```python
from build123d import *

# Parameters (mm, degrees)
SKETCH_W        = 56
SKETCH_H        = 56
PAD_DEPTH       = 18.68
PAD001_DEPTH    = 17
SKETCH004_W     = 50
SKETCH004_H     = 50
PAD002_DEPTH    = 3
SKETCH005_W     = 3.539247
SKETCH005_H     = 31.476045
SKETCH005_W_2   = 3.539498
SKETCH005_H_2   = 31.470025
POCKET003_DEPTH = 3
POCKET004_DEPTH = 5
POCKET005_DEPTH = 5
SKETCH003_W     = 10.900068
SKETCH003_H     = 5.909133
SKETCH003_W_2   = 10.899807
SKETCH003_H_2   = 5.880531
POCKET006_DEPTH = 10
POCKET007_DEPTH = 5
SKETCH002_W     = 7.004639
SKETCH002_H     = 5.993783
SKETCH002_W_2   = 50
SKETCH002_H_2   = 4
POCKET008_DEPTH = 5


with BuildPart() as part:
    # Sketch → Pad (new body)
    with BuildSketch(Plane.XY.offset(-11.59)):
        Rectangle(SKETCH_W, SKETCH_H)
        with BuildLine():
            Line((-21.013424, -25), (21.039206, -25))
            ThreePointArc((21.039206, -25), (23.83991, -23.83991), (25, -21.039206))
            Line((25, -21.039206), (25, 21.096275))
            Line((25, 21.096275), (25, 25))
            Line((21.096275, 25), (25, 25))
            Line((21.096275, 25), (-20.979066, 25))
            Line((-20.979066, 25), (-25, 25))
            Line((-25, 20.979066), (-25, 25))
            Line((-25, 20.979066), (-25, -21.013424))
            ThreePointArc((-25, -21.013424), (-23.832359, -23.832359), (-21.013424, -25))
        make_face(mode=Mode.SUBTRACT)
    extrude(amount=PAD_DEPTH)

    # Sketch → Pad001 (join)
    with BuildSketch(Plane.XY.offset(-11.59)):
        Rectangle(SKETCH_W, SKETCH_H)
        with BuildLine():
            Line((-21.013424, -25), (21.039206, -25))
            ThreePointArc((21.039206, -25), (23.83991, -23.83991), (25, -21.039206))
            Line((25, -21.039206), (25, 21.096275))
            Line((25, 21.096275), (25, 25))
            Line((21.096275, 25), (25, 25))
            Line((21.096275, 25), (-20.979066, 25))
            Line((-20.979066, 25), (-25, 25))
            Line((-25, 20.979066), (-25, 25))
            Line((-25, 20.979066), (-25, -21.013424))
            ThreePointArc((-25, -21.013424), (-23.832359, -23.832359), (-21.013424, -25))
        make_face(mode=Mode.SUBTRACT)
    extrude(amount=PAD001_DEPTH)

    # Sketch004 (on Sketch) → Pad002 (join)
    with BuildSketch(Plane.XY.offset(-11.59)):
        Rectangle(SKETCH004_W, SKETCH004_H)
    extrude(amount=PAD002_DEPTH)

    # Sketch005 (on Pad) → Pocket003 (cut)
    with BuildSketch(Plane.XY.offset(-11.59)):
        with Locations((-13.5995, -5.578318)):
            Rectangle(SKETCH005_W, SKETCH005_H)
        with Locations((13.600253, -5.565392)):
            Rectangle(SKETCH005_W_2, SKETCH005_H_2)
    extrude(amount=-POCKET003_DEPTH, mode=Mode.SUBTRACT)

    # Sketch005 (on Pad) → Pocket004 (cut)
    with BuildSketch(Plane.XY.offset(-11.59)):
        with Locations((-13.5995, -5.578318)):
            Rectangle(SKETCH005_W, SKETCH005_H)
        with Locations((13.600253, -5.565392)):
            Rectangle(SKETCH005_W_2, SKETCH005_H_2)
    extrude(amount=-POCKET004_DEPTH, mode=Mode.SUBTRACT)

    # Sketch005 (on Pad) → Pocket005 (cut)
    with BuildSketch(Plane.XY.offset(-11.59)):
        with Locations((-13.5995, -5.578318)):
            Rectangle(SKETCH005_W, SKETCH005_H)
        with Locations((13.600253, -5.565392)):
            Rectangle(SKETCH005_W_2, SKETCH005_H_2)
    extrude(amount=POCKET005_DEPTH, mode=Mode.SUBTRACT)

    # Sketch003 → Pocket006 (cut)
    with BuildSketch(Plane(origin=(25, 0, -3), x_dir=(0, 1, 0), z_dir=(1, 0, 0))):
        with Locations((-8.499979, 4.550172)):
            Rectangle(SKETCH003_W, SKETCH003_H)
        with Locations((8.599925, 4.534825)):
            Rectangle(SKETCH003_W_2, SKETCH003_H_2)
    extrude(amount=POCKET006_DEPTH, mode=Mode.SUBTRACT)

    # Sketch001 → Pocket007 (cut)
    with BuildSketch(Plane(origin=(10, 25, 0.26), x_dir=(1, 0, 0), z_dir=(0, -1, 0))):
        with BuildLine():
            Line((-3.099737, -3.5), (3.104045, -3.5))
            ThreePointArc((3.104045, -3.5), (5.505348, -2.505348), (6.5, -0.104045))
            Line((6.5, -0.104045), (6.5, 0.345505))
            ThreePointArc((6.5, 0.345505), (5.57607, 2.57607), (3.345505, 3.5))
            Line((3.345505, 3.5), (-3.100127, 3.5))
            ThreePointArc((-3.100127, 3.5), (-5.5042, 2.5042), (-6.5, 0.100127))
            Line((-6.5, 0.100127), (-6.5, -0.099737))
            ThreePointArc((-6.5, -0.099737), (-5.504086, -2.504086), (-3.099737, -3.5))
        make_face()
    extrude(amount=-POCKET007_DEPTH, mode=Mode.SUBTRACT)

    # Sketch002 → Pocket008 (cut)
    with BuildSketch(Plane(origin=(0, 25, -3), x_dir=(1, 0, 0), z_dir=(0, -1, 0))):
        with Locations((-8.503573, 4.513289)):
            Rectangle(SKETCH002_W, SKETCH002_H)
        with Locations((-0.011459, 8.993781)):
            Rectangle(SKETCH002_W_2, SKETCH002_H_2)
    extrude(amount=-POCKET008_DEPTH, mode=Mode.SUBTRACT)


solid = part.part
```
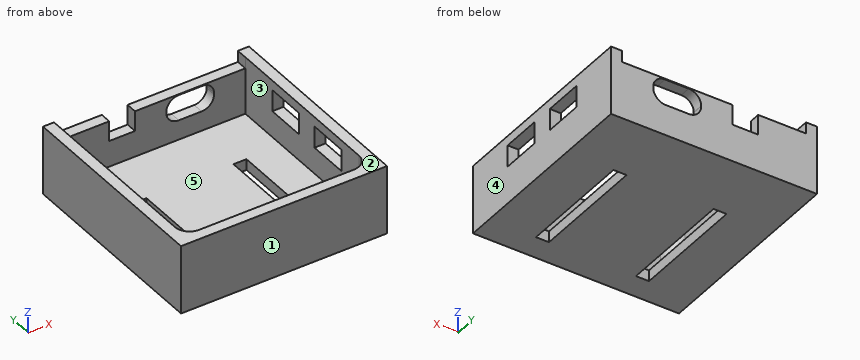
Input: part model. Units: mm. Frame: model coordinates. Face numbers are marked on the shaded views. A direction names the side the tool comes from. Round coordinates to 2 decimals unless told otherwise and drop trailing zeros. Loops run counter-clockwise (first coordinate to the right, second up) from the corner with the lowest first, then second, coordinate; pieces in that order, holes last. Notation, with made-up numbers: (32, -4.5) -> (37, -4.5) arc R27 cw to (37, 29.5) -> close; hole circle Ø11 at (63, -24). An arc over 180 degrees is marked (long way). Use one line per item in the form item = value. Start each with the question number.
Item 1: Section query D-D on y = 6. Return the cut outline in (x, z).
Item 2: Mould query, pull axis Y, two halves, no side actions, for the marked faces 1, 2 and 3. Classes: pulls with the +Y half, pulls with the -Y half, needs draft (parallel to the pull), parting line crosses it, or undercut.
Item 3: Material intervals for L1, parallel to Y at x = -20.5, z = -2; L2, parallel to X at y = -1, z = -10, sorted ascending. Write a range as from..to.
Item 4: Section query A-A on y = -16. Return the cut outline in (x, z).
Item 5: Contact query for flat-ended pins moving along their axis: pin 1 Ø8 at (x, y) = (-6, -22) entering from +Z; pin 2 Ø2.5 at (x, y) = (10, 27) entering from +Z; pin 3 Ø1 at (x, y) = (-13, -5) entering from +Z. Output: stop coordinate, or through.
Item 6: Section query C-C on z = -9.5. Return the cut outline in (x, y), then the cut area to 3 significant figures.
Item 7: Set-up query: the marked faces 4 and 5. Return all of +Z, -Z, +X, -X, +Y, -Y with unobstructed straight access to the full face (end or side cutting, diameter ignored); none if empty.
Item 8: Section query B-B on x = 8. Return the cut outline in (y, z), then the cut area to 3 significant figures.
Ans:
q1.outline = (-28, -11.59) -> (-15.37, -11.59) -> (-15.37, -8.59) -> (-25, -8.59) -> (-25, 7.09) -> (-28, 7.09) -> close; (-11.83, -11.59) -> (11.83, -11.59) -> (11.83, -8.59) -> (-11.83, -8.59) -> close; (15.37, -11.59) -> (28, -11.59) -> (28, -1.41) -> (25, -1.41) -> (25, -8.59) -> (15.37, -8.59) -> close; (25, 4.48) -> (28, 4.48) -> (28, 7.09) -> (25, 7.09) -> close
q2.face_1 = pulls with the -Y half
q2.face_2 = needs draft
q2.face_3 = undercut
q3.L1 = -28..-25, 25..28
q3.L2 = -28..-15.37, -11.83..11.83, 15.37..28
q4.outline = (-28, -11.59) -> (-15.37, -11.59) -> (-15.37, -8.59) -> (-25, -8.59) -> (-25, 7.09) -> (-28, 7.09) -> close; (-11.83, -11.59) -> (11.83, -11.59) -> (11.83, -8.59) -> (-11.83, -8.59) -> close; (15.37, -11.59) -> (28, -11.59) -> (28, 7.09) -> (25, 7.09) -> (25, -8.59) -> (15.37, -8.59) -> close
q5.pin_1 = 7.09
q5.pin_2 = 3.99
q5.pin_3 = through
q6.outline = (-28, -28) -> (28, -28) -> (28, 28) -> (-28, 28) -> close; hole (-15.37, -21.32) -> (-11.83, -21.32) -> (-11.83, 10.16) -> (-15.37, 10.16) -> close; hole (11.83, -21.3) -> (15.37, -21.3) -> (15.37, 10.17) -> (11.83, 10.17) -> close
q6.area = 2,910 mm^2
q7.face_4 = +Z, -Z, +X, +Y, -Y
q7.face_5 = +Z
q8.outline = (-28, -11.59) -> (28, -11.59) -> (28, -3.24) -> (25, -3.24) -> (25, -8.59) -> (-25, -8.59) -> (-25, 7.09) -> (-28, 7.09) -> close; (25, 3.76) -> (28, 3.76) -> (28, 3.99) -> (25, 3.99) -> close
q8.area = 232 mm^2
